Design review of the part built by this model. Coordinates are the model's own, in mm. Give positions to 0.01 mm unless a question says otherwise; leave off trailing zeros. Write each loop counter-clockwise with the first axis right and the second up, starting at its lowest first coordinate (ties: lowest second). Pieces come first, ordered by that corner, then holes. Notation, with made-up numbers: M 14,20 L 25,20 A7 cw 25,28 Z; hole C 88.5,43.25 d1. An arc over 180 degrees is marked long. Use a Markdown table: item, result. Add a question column.
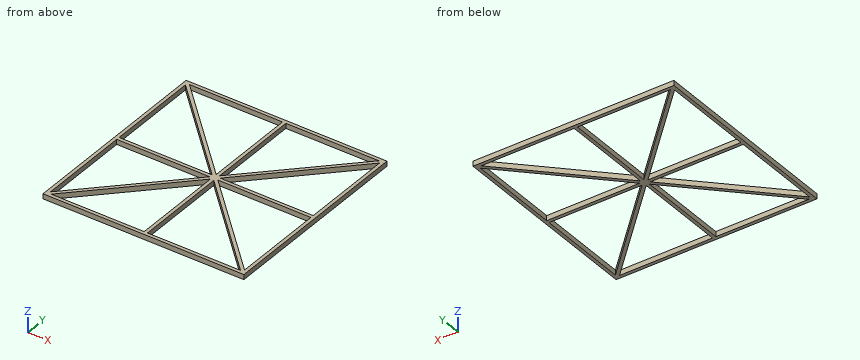
```python
from build123d import *

# Parameters (mm, degrees)
F0_W     = 120
F0_H     = 120
F1_DEPTH = 3


with BuildPart() as f1:
    # F0 (on Top) → F1 (new body)
    with BuildSketch(Plane.XY):
        Rectangle(F0_W, F0_H)
        Polygon((-1, -58), (-56.585786, -58), (-1, -2.414214), align=None, mode=Mode.SUBTRACT)
        Polygon((-58, -56.585786), (-58, -1), (-2.414214, -1), align=None, mode=Mode.SUBTRACT)
        Polygon((1, -58), (1, -2.414214), (56.585786, -58), align=None, mode=Mode.SUBTRACT)
        Polygon((58, -56.585786), (2.414214, -1), (58, -1), align=None, mode=Mode.SUBTRACT)
        Polygon((-58, 1), (-58, 56.585786), (-2.414214, 1), align=None, mode=Mode.SUBTRACT)
        Polygon((-1, 2.414214), (-56.585786, 58), (-1, 58), align=None, mode=Mode.SUBTRACT)
        Polygon((58, 1), (2.414214, 1), (58, 56.585786), align=None, mode=Mode.SUBTRACT)
        Polygon((1, 2.414214), (1, 58), (56.585786, 58), align=None, mode=Mode.SUBTRACT)
    extrude(amount=F1_DEPTH)


solid = f1.part
```
(1) Wall thickness on L1, parallel to Y at x = 31.5, z = 1.75; L2, parallel to X at y = 54, z = 2.85; L3, parallel to Y at x = -11, z = 2.7: over which ranges is each line inside the solid? List them lowest first.
(2) Add section A-A on y = 5. Give the boundary of the cut face in (x, z), then the cut area to 3 significant figures.
(3) Add section B-B on x = -6. Give the boundary of the cut face in (y, z).
(4) Add section C-C on z = 1.35. Give the number of separate pieces and of enclosed holes in the cut face, then the cut area to 3 significant figures.
(5) For pin 1 (8 mm diameter, centred on x = -13, y = 0, fed in from -Z), flat-tipped, find the tip position at first contact; note if it passes through.
From the geometry:
| question | item | result |
|---|---|---|
| 1 | L1 | y = -60 to -58, -32.91 to -30.09, -1 to 1, 30.09 to 32.91, 58 to 60 |
| 1 | L2 | x = -60 to -58, -55.41 to -52.59, -1 to 1, 52.59 to 55.41, 58 to 60 |
| 1 | L3 | y = -60 to -58, -12.41 to -9.59, -1 to 1, 9.59 to 12.41, 58 to 60 |
| 2 | outline | M -60,0 L -58,0 L -58,3 L -60,3 Z; M -6.41,0 L -3.59,0 L -3.59,3 L -6.41,3 Z; M -1,0 L 1,0 L 1,3 L -1,3 Z; M 3.59,0 L 6.41,0 L 6.41,3 L 3.59,3 Z; M 58,0 L 60,0 L 60,3 L 58,3 Z |
| 2 | area | 35.0 mm^2 |
| 3 | outline | M -60,0 L -58,0 L -58,3 L -60,3 Z; M -7.41,0 L -4.59,0 L -4.59,3 L -7.41,3 Z; M -1,0 L 1,0 L 1,3 L -1,3 Z; M 4.59,0 L 7.41,0 L 7.41,3 L 4.59,3 Z; M 58,0 L 60,0 L 60,3 L 58,3 Z |
| 4 | separate pieces | 1 |
| 4 | enclosed holes | 8 |
| 4 | area | 2,040 mm^2 |
| 5 | pin 1 | stops at z = 0 |
